```python
from build123d import *

# Parameters (mm, degrees)
F0_W     = 30
F0_H     = 3
F1_DEPTH = 3
F2_W     = 3.1
F2_H     = 25
F3_DEPTH = 25
F5_DEPTH = 25
F6_W     = 3
F6_H     = 30
F7_DEPTH = 25


with BuildPart() as f1:
    # F0 (on Right) → F1 (new body)
    with BuildSketch(Plane.YZ):
        Polygon((-45.8, 83), (-45.8, 6.5), (-48.823975, 6.5), (-48.823975, 0), (-45.8, -60.5), (-13.3, -60.5), (16.7, -60.5), (49.2, -60.5), (49.2, -35.5), (73.2, -35.5), (73.2, 6.5), (49.2, 6.5), (49.2, 83), align=None)
        with Locations((1.7, -62)):
            Rectangle(F0_W, F0_H)
    extrude(amount=F1_DEPTH)

    # F2 (on face) → F3 (cut)
    with BuildSketch(Plane.YZ.offset(3)):
        with Locations((61.65, -14.5)):
            Rectangle(F2_W, F2_H)
    extrude(amount=-F3_DEPTH, mode=Mode.SUBTRACT)

    # F4 (on face) → F5 (cut)
    with BuildSketch(Plane.YZ.offset(3)):
        with BuildLine():
            Line((31.499346, -28.6), (-20.500654, -28.6))
            ThreePointArc((-20.500654, -28.6), (-23.329081, -29.771573), (-24.500654, -32.6))
            Line((-24.500654, -32.6), (-24.500654, -34.4))
            ThreePointArc((-24.500654, -34.4), (-23.329081, -37.228427), (-20.500654, -38.4))
            Line((-20.500654, -38.4), (31.499346, -38.4))
            ThreePointArc((31.499346, -38.4), (34.327773, -37.228427), (35.499346, -34.4))
            Line((35.499346, -34.4), (35.499346, -32.6))
            ThreePointArc((35.499346, -32.6), (34.327773, -29.771573), (31.499346, -28.6))
        make_face()
    extrude(amount=-F5_DEPTH, mode=Mode.SUBTRACT)

    # F6 (on face) → F7 (cut)
    with BuildSketch(Plane.YZ.offset(3)):
        with Locations((-44.3, 43)):
            Rectangle(F6_W, F6_H)
        with Locations((47.7, 43)):
            Rectangle(F6_W, F6_H)
    extrude(amount=-F7_DEPTH, mode=Mode.SUBTRACT)


solid = f1.part
```
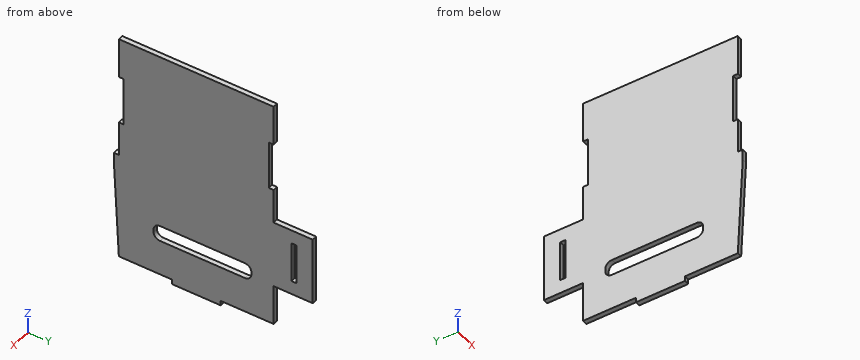
Read the model definition and answer for the solid it produces. Units are mm, in the model's axes. Coordinates: 2 decimals unless noted, no trailing zeros. Loops run counter-clockwise (first coordinate to the right, second up) from the corner with the lowest first, then second, coordinate; pieces in that order, holes last.
(1) Flat-ended cylindrical pins translate along their axes: pin 1 Ø1.5 at (x, z) = (1.5, 41.5) entering from +Y; pin 2 Ø1.5 at (x, y) = (1, -30) entering from -Z; pin 3 Ø0.9 at (x, z) = (2, 13.5) entering from -Y. Find the tip coordinate at first contact, or state that the pin passes through.
Solution:
pin 1: stops at y = 46.2
pin 2: stops at z = -60.5
pin 3: stops at y = -45.8
(2) Consider line 1 along Z through (x, y) = (1.25, -6); line 2 along Z through (x, y) = (2.55, -29); line 3 along Y through (x, z) = (1.95, 16.5). Determine where each line is inside the solid, lowest interval first.
Solution:
line 1: z = -63.5 to -38.4, -28.6 to 83
line 2: z = -60.5 to 83
line 3: y = -45.8 to 49.2
(3) The part is cut by section A-A (y = -15). Determine the outline of the cut face in (x, z), and give its area (3 significant figures).
Solution:
outline: (0, -60.5) - (3, -60.5) - (3, -38.4) - (0, -38.4) - close; (0, -28.6) - (3, -28.6) - (3, 83) - (0, 83) - close
area: 401 mm2
(4) The part is cut by section B-B (x = 0.9). Count the separate pieces of the cut face and the enclosed holes in it, and give its area (3 significant figures).
Solution:
separate pieces: 1
enclosed holes: 2
area: 14,000 mm2
(5) The part is cut by section C-C (z = 47.5). Determine the outline of the cut face in (x, y), and give its area (3 significant figures).
Solution:
outline: (0, -42.8) - (3, -42.8) - (3, 46.2) - (0, 46.2) - close
area: 267 mm2
(6) The part is cut by section D-D (z = 10.5). Determine the outline of the cut face in (x, y).
Solution:
outline: (0, -45.8) - (3, -45.8) - (3, 49.2) - (0, 49.2) - close
